Read the model definition and answer for the solid it produces. Units are mm, in the model's axes. A direction names the side the tool comes from. Give positions to 0.01 mm unless a question says otherwise; leave off trailing zeros. Write each loop counter-clockwise with the first axis right and the second up, starting at its lowest first coordinate (ties: lowest second). Pieces come first, ordered by that corner, then holes. Notation, with made-up numbers: (-8.75, 55) - (36.25, 55) arc R21 ccw to (36.25, 75) - close; hole circle Ø1 at (-39, -36). An arc over 180 degrees is marked (long way). Answer as CSV lines item,"result".
```python
from build123d import *

# Parameters (mm, degrees)
F0_R          = 24.765
F0_R_2        = 21.082
F1_DEPTH      = 59.055
F2_R          = 24.765
F2_R_2        = 21.082
F3_DEPTH      = 59.055
F4_R          = 24.765
F4_R_2        = 21.082
F5_DEPTH      = 59.055
F6_DEPTH      = 59.0560001
F7_DEPTH      = 59.0560001
F8_DEPTH      = 59.0560001
F8_DEPTH_BACK = 59.0560001
F9_SIZE2      = 4.7397045256
F9_SIZE       = 1.27
F9_2_SIZE2    = 4.7397045256
F9_2_SIZE     = 1.27
F9_3_SIZE2    = 4.7397045256
F9_3_SIZE     = 1.27
F10_SIZE2     = 4.7397045256
F10_SIZE      = 1.27


with BuildPart() as f1:
    # F0 (on Front) → F1 (new body, symmetric)
    with BuildSketch(Plane.XZ):
        Circle(F0_R)
        Circle(F0_R_2, mode=Mode.SUBTRACT)
    extrude(amount=F1_DEPTH, both=True)

    # F2 (on Top) → F3 (join)
    with BuildSketch(Plane.XY):
        Circle(F2_R)
        Circle(F2_R_2, mode=Mode.SUBTRACT)
    extrude(amount=F3_DEPTH)

    # F4 (on Right) → F5 (join)
    with BuildSketch(Plane.YZ):
        Circle(F4_R)
        Circle(F4_R_2, mode=Mode.SUBTRACT)
    extrude(amount=F5_DEPTH)

    # F4 (on Right) → F6 (cut, through all)
    with BuildSketch(Plane.YZ):
        Circle(F4_R_2)
    extrude(amount=F6_DEPTH, mode=Mode.SUBTRACT)

    # F2 (on Top) → F7 (cut, through all)
    with BuildSketch(Plane.XY):
        Circle(F2_R_2)
    extrude(amount=F7_DEPTH, mode=Mode.SUBTRACT)

    # F0 (on Front) → F8 (cut, two sides)
    with BuildSketch(Plane.XZ) as f8_sk:
        Circle(F0_R_2)
    extrude(amount=F8_DEPTH, mode=Mode.SUBTRACT)
    extrude(f8_sk.sketch, amount=-F8_DEPTH_BACK, mode=Mode.SUBTRACT)

    # F9
    f9_edges = [f1.edges().sort_by_distance(p)[0] for p in [
        (-24.765, 0, 59.055),
    ]]
    f9_side = f1.faces().sort_by_distance((-24.06454, 0, 59.055))[0]
    chamfer(f9_edges, length=F9_SIZE, length2=F9_SIZE2, reference=f9_side)

    # F9#2
    f9_2_edges = [f1.edges().sort_by_distance(p)[0] for p in [
        (-24.765, -59.055, 0),
    ]]
    f9_2_side = f1.faces().sort_by_distance((-24.06454, -59.055, 0))[0]
    chamfer(f9_2_edges, length=F9_2_SIZE, length2=F9_2_SIZE2, reference=f9_2_side)

    # F9#3
    f9_3_edges = [f1.edges().sort_by_distance(p)[0] for p in [
        (59.055, -24.765, 0),
    ]]
    f9_3_side = f1.faces().sort_by_distance((59.055, -24.06454, 0))[0]
    chamfer(f9_3_edges, length=F9_3_SIZE, length2=F9_3_SIZE2, reference=f9_3_side)

    # F10
    f10_edges = [f1.edges().sort_by_distance(p)[0] for p in [
        (-24.765, 59.055, 0),
    ]]
    f10_side = f1.faces().sort_by_distance((-24.06454, 59.055, 0))[0]
    chamfer(f10_edges, length=F10_SIZE, length2=F10_SIZE2, reference=f10_side)


solid = f1.part
```
(1) The mould has two halves that part along Z. Classify faces 6 (the cylindrical face through (-4.57, 0.83, -20.58)), 7 (the cylindrical face through (-24.74, 1.09, 38.85)), 8 (the conical face through (58.759, -5.11, -23.014)), 9 (the cylindrical face through (35.68, -4.57, -20.58)): +Z half, -Z half, draft (parallel to the pull), parting line (faces both ways), or undercut.
Worked out:
face 6,"undercut"
face 7,"draft"
face 8,"parting line"
face 9,"undercut"
(2) A cutting plane is placed at B-B (x = 51). Write down the section's boundary in (y, z) (3 decimals), and give its area (3 significant figures).
Worked out:
outline,"circle Ø49.53 at (0, 0); hole circle Ø42.164 at (0, 0)"
area,"530 mm^2"
(3) A cutting plane is placed at D-D (z = 5.5). Count the separate pieces of the cut face and the enclosed holes in it, and give its area (3 significant figures).
Worked out:
separate pieces,"3"
enclosed holes,"0"
area,"987 mm^2"
(4) Find the intervals of material crossed by L1, parallel to Z at x = -1, y = 22.5 (3 decimals); L2, parallel to Z at x = 26, y = 0 (3 decimals), in increasing order.
Worked out:
L1,"z = -24.745 to -21.058, 21.058 to 59.055"
L2,"z = -24.765 to -21.082, 21.082 to 24.765"
(5) For faces 1 (the cylindrical face through (-21.06, 0.93, 35.68)), 2 (the conical face through (-5.11, -58.759, -23.014)), 3 (the cylindrical face through (38.848, -5.369, -24.176)), 4 (the cylindrical face through (-19.65, -0.76, -15.07)), 5 (the flat face through (-4, -21, 59.055)), determine the directions among +Z, -Z, +X, -X, +Y, -Y from which every point of the face is accessible in a straight line to the end or side of a thin tool.
Worked out:
face 1,"+Z"
face 2,"-Y"
face 3,"+X"
face 4,"none"
face 5,"+Z, +X, -X, +Y, -Y"
(6) A cutting plane is placed at A-A (y = 0). Write down the section's boundary in (x, z) (3 decimals), and give its area (3 significant figures).
Worked out:
outline,"(-24.765, 0) arc R24.765 ccw to (0, -24.765) - (54.315, -24.765) - (59.055, -23.495) - (59.055, -21.082) - (0, -21.082) arc R21.082 cw to (-21.082, 0) - (-21.082, 59.055) - (-23.495, 59.055) - (-24.765, 54.315) - close; (21.082, 21.082) - (59.055, 21.082) - (59.055, 23.495) - (54.315, 24.765) - (24.765, 24.765) - (24.765, 54.315) - (23.495, 59.055) - (21.082, 59.055) - close"
area,"822 mm^2"
(7) Each of these flat-tipped pins is pushed along its axis until it touches: P1, Ø3, axis at x = 7, y = -6, coming from the +Z side; P2, Ø5, axis at x = 23, z = -5, coming from the +Y side (3 decimals); P3, Ø1, axis at x = 44, y = 15, coming from the +Z side; P4, Ø1, axis at x = 23, y = 19.5, coming from the +Z side. Where does it stop, or does it pass through?
Worked out:
P1,"stops at z = -19.73"
P2,"stops at y = 59.055"
P3,"stops at z = 20.08"
P4,"stops at z = 15.88"
